from build123d import *

# Parameters (mm, degrees)
SKETCH_1_W                                          = 70
SKETCH_1_H                                          = 140
BASE_70X140X5_DEPTH                                 = 5
CHASSIS_ADJUSTMENT_SLOTS_UNVERIFIED_POSI_DEPTH      = 79.421935707
CHASSIS_ADJUSTMENT_SLOTS_UNVERIFIED_POSI_DEPTH_BACK = 79.421935707
SKETCH_2_W                                          = 3.4
SKETCH_2_H                                          = 12
SUPPORT_AND_SERVO_MOUNT_M3_CLEARANCE_DEPTH          = 79.421935707
SUPPORT_AND_SERVO_MOUNT_M3_CLEARANCE_DEPTH_BACK     = 79.421935707
SKETCH_3_R                                          = 1.7


with BuildPart() as part:
    # 草图1 → Base_70x140x5 (new body)
    with BuildSketch(Plane.XY):
        Rectangle(SKETCH_1_W, SKETCH_1_H)
    extrude(amount=BASE_70X140X5_DEPTH)

    # 草图2 → Chassis_adjustment_slots_UNVERIFIED_positions (cut, two sides: drawn at the far end of the back side and taken through both)
    with BuildSketch(Plane.XY.offset(-CHASSIS_ADJUSTMENT_SLOTS_UNVERIFIED_POSI_DEPTH_BACK)):
        with Locations((-26, -51)):
            Rectangle(SKETCH_2_W, SKETCH_2_H)
        with Locations((-26, 51)):
            Rectangle(SKETCH_2_W, SKETCH_2_H)
        with Locations((26, -51)):
            Rectangle(SKETCH_2_W, SKETCH_2_H)
        with Locations((26, 51)):
            Rectangle(SKETCH_2_W, SKETCH_2_H)
    extrude(amount=CHASSIS_ADJUSTMENT_SLOTS_UNVERIFIED_POSI_DEPTH + CHASSIS_ADJUSTMENT_SLOTS_UNVERIFIED_POSI_DEPTH_BACK, mode=Mode.SUBTRACT)

    # 草图3 → Support_and_servo_mount_M3_clearance (cut, two sides: drawn at the far end of the back side and taken through both)
    with BuildSketch(Plane.XY.offset(-SUPPORT_AND_SERVO_MOUNT_M3_CLEARANCE_DEPTH_BACK)):
        with Locations((-20, -14)):
            Circle(SKETCH_3_R)
        with Locations((-20, 14)):
            Circle(SKETCH_3_R)
        with Locations((20, -14)):
            Circle(SKETCH_3_R)
        with Locations((20, 14)):
            Circle(SKETCH_3_R)
        with Locations((-9, 57)):
            Circle(SKETCH_3_R)
        with Locations((-9, 66)):
            Circle(SKETCH_3_R)
        with Locations((31, 57)):
            Circle(SKETCH_3_R)
        with Locations((31, 66)):
            Circle(SKETCH_3_R)
    extrude(amount=SUPPORT_AND_SERVO_MOUNT_M3_CLEARANCE_DEPTH + SUPPORT_AND_SERVO_MOUNT_M3_CLEARANCE_DEPTH_BACK, mode=Mode.SUBTRACT)


solid = part.part
Input: part model. Units: mm. Frame: model coordinates. A direction names the side the tool comes from. Coordinates: 2 decimals unless noted, no trailing zeros. Loops run counter-clockwise (first coordinate to the right, second up) from the corner with the lowest first, then second, coordinate; pieces in that order, holes last.
(1) Section B-B on y = 66. Return the cut outline in (x, z).
(2) Pull-direction query (X, two-part tool) for faces 1 (the face through (0, -70, 2)), 2 (the face through (26, 45, 2)), 3 (the face through (-10.35, 64.97, 2.47)); classes: released by +X, released by -X, zero draft, split by the parting line, or undercut.
(3) Section C-C on z = 3.15. Count the separate pieces of the cut face and the enclosed holes in it, then the cut area to 3 significant figures.
(4) Material intervals for probe 1 along X at (y, z) = (66, 2.8); probe 2 along Y at (x, z) = (-20, 2.65); probe 3 along Y at (x, z) = (31, 2.55), sorted ascending.
(5) Set-up query: faces 4 (the face through (24.3, -51, 2)), 5 (the face through (0, 1, 0)). Return all of +Z, -Z, +X, -X, +Y, -Y with unobstructed straight access to the full face (end or side cutting, diameter ignored); none if empty.
(6) Section A-A on x = -20. Return the cut outline in (y, z).
(7) First-contact query: pin 1 Ø4 at (x, y) = (20, 14) entering from -Z. Flat tip, straight axial feed; report the tip coordinate or a pass-through.
Data:
1. outline: (-35, 0) - (-10.7, 0) - (-10.7, 5) - (-35, 5) - close; (-7.3, 0) - (29.3, 0) - (29.3, 5) - (-7.3, 5) - close; (32.7, 0) - (35, 0) - (35, 5) - (32.7, 5) - close
2. face 1: zero draft
2. face 2: undercut
2. face 3: undercut
3. separate pieces: 1
3. enclosed holes: 12
3. area: 9,560 mm2
4. probe 1: x = -35 to -10.7, -7.3 to 29.3, 32.7 to 35
4. probe 2: y = -70 to -15.7, -12.3 to 12.3, 15.7 to 70
4. probe 3: y = -70 to 55.3, 58.7 to 64.3, 67.7 to 70
5. face 4: +Z, -Z
5. face 5: -Z, +X, -X, +Y, -Y
6. outline: (-70, 0) - (-15.7, 0) - (-15.7, 5) - (-70, 5) - close; (-12.3, 0) - (12.3, 0) - (12.3, 5) - (-12.3, 5) - close; (15.7, 0) - (70, 0) - (70, 5) - (15.7, 5) - close
7. pin 1: stops at z = 0
